```python
from build123d import *

# Parameters (mm, degrees)
SKETCH1_W           = 40
SKETCH1_H           = 50
BOSS_EXTRUDE1_DEPTH = 5
SKETCH2_W           = 5
SKETCH2_H           = 50
BOSS_EXTRUDE2_DEPTH = 25
SKETCH3_R           = 4
CUT_EXTRUDE1_DEPTH  = 56.901699437
SKETCH4_W           = 5
SKETCH4_H           = 30
BOSS_EXTRUDE3_DEPTH = 20
SKETCH5_R           = 3
BOSS_EXTRUDE4_DEPTH = 5
SKETCH6_R           = 15
BOSS_EXTRUDE5_DEPTH = 30


with BuildPart() as part:
    # Sketch1 → Boss-Extrude1 (new body)
    with BuildSketch(Plane.XY):
        Rectangle(SKETCH1_W, SKETCH1_H)
    extrude(amount=BOSS_EXTRUDE1_DEPTH)

    # Sketch2 → Boss-Extrude2 (add)
    with BuildSketch(Plane.XY.offset(5)):
        with Locations((-17.5, 0)):
            Rectangle(SKETCH2_W, SKETCH2_H)
        with Locations((17.5, 0)):
            Rectangle(SKETCH2_W, SKETCH2_H)
    extrude(amount=BOSS_EXTRUDE2_DEPTH)

    # Sketch3 → Cut-Extrude1 (cut, through all)
    with BuildSketch(Plane.ZY.offset(20)):
        with Locations((20, 0)):
            Circle(SKETCH3_R)
    extrude(amount=-CUT_EXTRUDE1_DEPTH, mode=Mode.SUBTRACT)

    # Sketch4 → Boss-Extrude3 (add)
    with BuildSketch(Plane.ZY.offset(20)):
        with Locations((2.5, 0)):
            Rectangle(SKETCH4_W, SKETCH4_H)
    extrude(amount=BOSS_EXTRUDE3_DEPTH)

    # Sketch5 → Boss-Extrude4 (add)
    with BuildSketch(Plane.XY.offset(5)):
        with BuildLine():
            Line((-40, 15), (-40, -15))
            Line((-40, -15), (-91.641900121, 52.474794317))
            ThreePointArc((-91.641900121, 52.474794317), (-90.399583659, 62.866857636), (-79.978416938, 61.898552722))
            Line((-79.978416938, 61.898552722), (-40, 15))
        make_face()
        with Locations((-85.686070809, 57.033094132)):
            Circle(SKETCH5_R, mode=Mode.SUBTRACT)
    extrude(amount=-BOSS_EXTRUDE4_DEPTH)

    # Sketch6 → Boss-Extrude5 (add)
    with BuildSketch(Plane(origin=(0, 0, 0), x_dir=(-1, 0, 0), z_dir=(0, 0, -1))):
        Circle(SKETCH6_R)
    extrude(amount=BOSS_EXTRUDE5_DEPTH)


solid = part.part
```
Can you work these out from the model? Positions are in its coordinate system, mm. A direction names the side the tool comes from. Round coordinates to 2 decimals unless told otherwise and drop trailing zeros. Loops run counter-clockwise (first coordinate to the right, second up) from the corner with the lowest first, then second, coordinate; pieces in that order, holes last.
Item 1: Which directions (+Z, -Z, +X, -X, +Y, -Y) give clear straight access to the entire face, cutting with the end or side of a thin tool? Please do faces 4 (the flat face through (-30, 15, 2)), 5 (the flat face through (0, 0, 5)), 6 (the cylindrical face through (14.985, 0.66, -14.79)), 7 (the flat face through (-54, 22, 5)), 8 (the flat face through (-0.3, 25, 4.8)).
Item 2: Suppose I cut it at A-A, the plane z = 20. Write out the boundary of the cut face in (x, y), then the cut area to 3 significant figures.
Item 3: Please list where these lines run through material, in increasing order: L1, parallel to Y at x = 16.65, z = 20; L2, parallel to X at y = 6, z = 16.5; L3, parallel to Z at x = -11.5, y = -10.5.
Item 4: Will these pins go through, and if not, where does the flat tip stop? pin 1 Ø12 at (x, y) = (-57.5, 26) entering from -Z; pin 2 Ø8 at (y, z) = (40, 1.5) entering from +X; pin 3 Ø15 at (x, y) = (1.5, -11) entering from +Z.
Item 5: Suppose I cut it at B-B, the plane y = 0. Write out the boundary of the cut face in (x, z), then the cut area to 3 significant figures.
Item 6: If we mould it in two halves opening along X, with no side actions, what happens to faces 1 (the cylindrical face through (-90.525, 62.764, 2.535)), 2 (the cylindrical face through (17.5, -2.4, 16.8)), 3 (the flat face through (15, 0, 15))? For each: +X half, -X half, draft (parallel to the pull), parting line (faces both ways), or undercut.
Item 7: Suppose I cut it at D-D, the plane x = 0. Write out the boundary of the cut face in (y, z), then the cut area to 3 significant figures.
Item 8: Suppose I cut it at C-C, the plane y = -18. Write out the boundary of the cut face in (x, z), then the cut area to 3 significant figures.
Reported:
1. face 4: +Z, -Z, +Y
1. face 5: +Z, +Y, -Y
1. face 6: -Z
1. face 7: +Z, -X, +Y, -Y
1. face 8: +Z, -Z, +X, +Y
2. outline: (-20, -25) - (-15, -25) - (-15, -4) - (-20, -4) - close; (-20, 4) - (-15, 4) - (-15, 25) - (-20, 25) - close; (15, -25) - (20, -25) - (20, -4) - (15, -4) - close; (15, 4) - (20, 4) - (20, 25) - (15, 25) - close
2. area: 420 mm2
3. L1: y = -25 to -4, 4 to 25
3. L2: x = -20 to -15, 15 to 20
3. L3: z = 0 to 5
4. pin 1: stops at z = 0
4. pin 2: stops at x = -57.9
4. pin 3: stops at z = 5
5. outline: (-51.48, 0) - (-15, 0) - (-15, -30) - (15, -30) - (15, 0) - (20, 0) - (20, 16) - (15, 16) - (15, 5) - (-15, 5) - (-15, 16) - (-20, 16) - (-20, 5) - (-51.48, 5) - close; (-20, 24) - (-15, 24) - (-15, 30) - (-20, 30) - close; (15, 24) - (20, 24) - (20, 30) - (15, 30) - close
5. area: 1,430 mm2
6. face 1: parting line
6. face 2: draft
6. face 3: undercut
7. outline: (-25, 0) - (-15, 0) - (-15, -30) - (15, -30) - (15, 0) - (25, 0) - (25, 5) - (-25, 5) - close
7. area: 1,150 mm2
8. outline: (-20, 0) - (20, 0) - (20, 30) - (15, 30) - (15, 5) - (-15, 5) - (-15, 30) - (-20, 30) - close
8. area: 450 mm2
